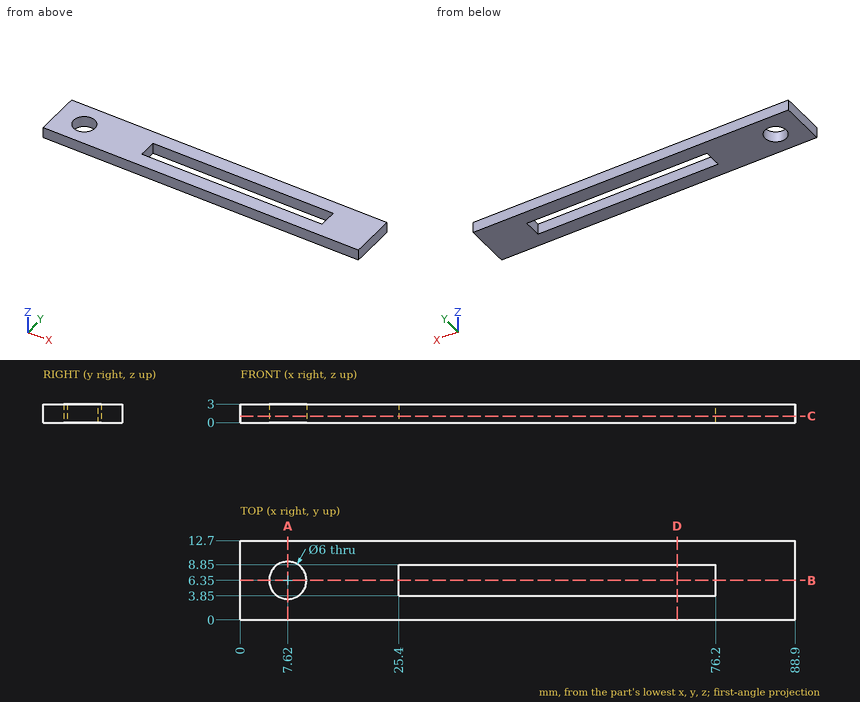
Design review of the part shown in the three views and the two pictorial views. Dimensions are in mm from the part's minimum x, y and z. Round coordinates to 2 decimals unless told otherwise and drop trailing zeros. Write each loop counter-clockwise with the first axis right and the second up, starting at its lowest first coordinate (ties: lowest second). Pieces come first, ordered by that corner, then holes. Notation, with made-up numbers: (-27, -27.5) -> (-22, -27.5) arc R17 ccw to (-22, -16.5) -> close; hole circle Ø11 at (87.5, 62). An arc over 180 degrees is marked (long way). One line per question, with ' | ' between items. Start each with the question number.
1) Add section B-B (y = 6.35). Write out the cut boundary in (x, z), and give its area (3 significant figures).
2) Add section D-D (x = 70). Write out the cut boundary in (y, z).
3) Add section C-C (z = 1.05). Write out the cut boundary in (x, y).
4) Add section A-A (x = 7.62). Write out the cut boundary in (y, z).
5) Wall thickness on line 1 along X through (y, z) = (6.5, 2.75); line 2 along X through (y, z) = (7.5, 0.1); line 3 along Y through (x, z) = (47.5, 1.55): over which ranges is each line inside the solid? List them lowest first.
Reported:
1) outline: (0, 0) -> (4.62, 0) -> (4.62, 3) -> (0, 3) -> close; (10.62, 0) -> (25.4, 0) -> (25.4, 3) -> (10.62, 3) -> close; (76.2, 0) -> (88.9, 0) -> (88.9, 3) -> (76.2, 3) -> close | area: 96.3 mm²
2) outline: (0, 0) -> (3.85, 0) -> (3.85, 3) -> (0, 3) -> close; (8.85, 0) -> (12.7, 0) -> (12.7, 3) -> (8.85, 3) -> close
3) outline: (0, 0) -> (88.9, 0) -> (88.9, 12.7) -> (0, 12.7) -> close; hole circle Ø6 at (7.62, 6.35); hole (25.4, 3.85) -> (76.2, 3.85) -> (76.2, 8.85) -> (25.4, 8.85) -> close
4) outline: (0, 0) -> (3.35, 0) -> (3.35, 3) -> (0, 3) -> close; (9.35, 0) -> (12.7, 0) -> (12.7, 3) -> (9.35, 3) -> close
5) line 1: x = 0 to 4.62, 10.62 to 25.4, 76.2 to 88.9 | line 2: x = 0 to 4.85, 10.39 to 25.4, 76.2 to 88.9 | line 3: y = 0 to 3.85, 8.85 to 12.7
